```python
from build123d import *

# Parameters (mm, degrees)
F_10_0_1935_DIAMETER_HOLE1_D     = 4.9149
F_33_64_0_51563_DIAMETER_HOLE1_D = 13.097002


with BuildPart() as part:
    # Sketch1 → Revolve1 (revolve)
    with BuildSketch(Plane.XY):
        Polygon((-3.175, -19.05), (-12.7, -19.05), (-12.7, -38.1), align=None)
        Polygon((-12.7, -38.1), (-12.7, -19.05), (-3.175, -19.05), (-3.175, 0), (-15.875, 0), (-15.875, -19.05), (-31.75, -19.05), (-31.75, -38.1), (-23.8125, -38.1), (-23.8125, -34.9631), (-19.0373, -34.9631), (-19.0373, -38.1), align=None)
    revolve(axis=Axis((0, 0, 0), (0, -1, 0)))

    # #10 (0.1935) Diameter Hole1 (through all)
    with Locations(Plane(origin=(0, 0, 0), x_dir=(1, 0, 0), z_dir=(0, 1, 0))):
        with Locations((19.083044257, 19.083044257), (-19.083044257, 19.083044257), (-19.083044257, -19.083044257), (19.083044257, -19.083044257)):
            Hole(F_10_0_1935_DIAMETER_HOLE1_D / 2)

    # 33/64 (0.51563) Diameter Hole1 (through all)
    with Locations(Plane(origin=(0, 0, 0), x_dir=(1, 0, 0), z_dir=(0, 1, 0))):
        with Locations((0, 0)):
            Hole(F_33_64_0_51563_DIAMETER_HOLE1_D / 2)


solid = part.part
```
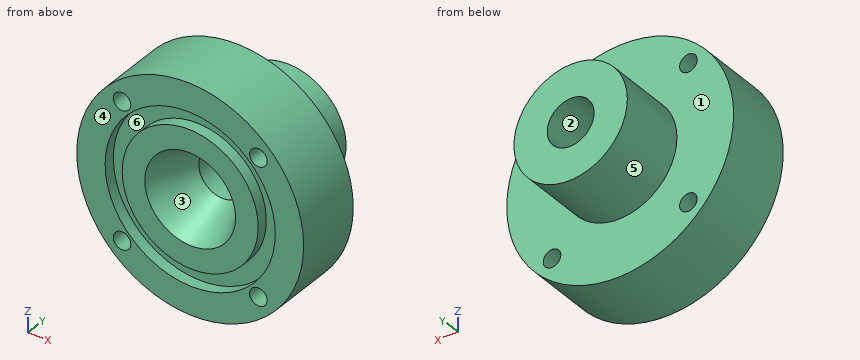
Here's how the part is built. I have some questions about the finished solid (model axes, mm). Face numbers are marked on the shaded views. A direction names the side the tool comes from. Coordinates: 2 decimals unless noted, no trailing zeros. Order: outer loops, then holes, each group sorted by start corner. A loop starts at its lowest first (then second) coordinate and runs counter-clockwise, first axis right, second up.
1) We'd pull the mould along X, two halves only. Please class the marked faces 3, 4, 5 and 6: +X half, -X half, draft (parallel to the pull), parting line (faces both ways), or undercut.
2) Which directions (+Z, -Z, +X, -X, +Y, -Y) give clear straight access to the entire face, cutting with the end or side of a thin tool? Please do the marked faces 1 and 2.
3) Imagine slicing it at D-D on y = -20.5. List the corners of the cut face in (x, z) for me, and give its area (3 significant figures).
4) Will these pins go through, and if not, where does the flat tip stop? pin 1 (1 mm diameter, centred on x = -6, y = -12.5, fed in from -Z); pin 2 (2 mm diameter, centred on x = -13, y = -18.5, fed in from +Z); pin 3 (1 mm diameter, centred on x = 10.5, y = -12.5, fed in from -Z).
5) I need wall thicknesses on line 1 (Z direction, x = 0, y = -35); line 2 (X direction, y = -22, z = 17); line 3 (X direction, y = -36.6, z = 0). Which ranges of each line are inside material? Lowest first, please.
Response values:
1. face 3: undercut
1. face 4: draft
1. face 5: parting line
1. face 6: undercut
2. face 1: +Y
2. face 2: +Y, -Y
3. outline: circle Ø63.5 at (0, 0); hole circle Ø4.91 at (-19.08, -19.08); hole circle Ø4.91 at (-19.08, 19.08); hole circle Ø13.1 at (0, 0); hole circle Ø4.91 at (19.08, -19.08); hole circle Ø4.91 at (19.08, 19.08)
3. area: 2,960 mm2
4. pin 1: stops at z = -14.89
4. pin 2: stops at z = 29.33
4. pin 3: stops at z = -12.33
5. line 1: z = -31.75 to -23.81, -19.04 to -11.15, 11.15 to 19.04, 23.81 to 31.75
5. line 2: x = -26.82 to -20.39, -17.78 to 17.78, 20.39 to 26.82
5. line 3: x = -31.75 to -23.81, -19.04 to -11.95, 11.95 to 19.04, 23.81 to 31.75
